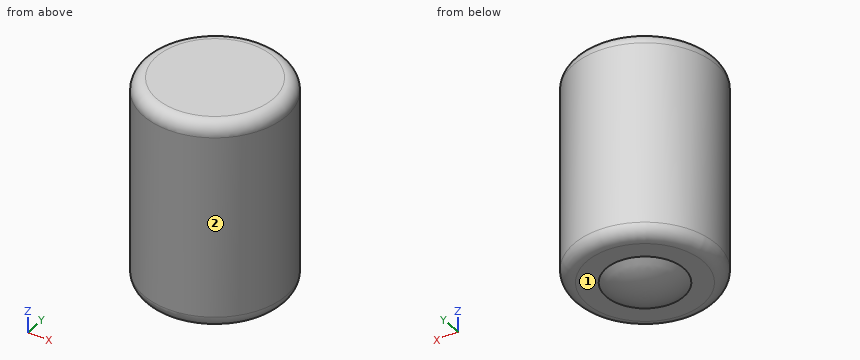
from build123d import *

# Parameters (mm, degrees)
F0_R     = 5.5
F1_DEPTH = 16
F2_R     = 1
F3_T     = -1.5
F6_R     = 1


with BuildPart() as f1:
    # F0 (on Top) → F1 (new body)
    with BuildSketch(Plane.XY):
        Circle(F0_R)
    extrude(amount=-F1_DEPTH)

    # F2
    f2_edges = [f1.edges().sort_by_distance(p)[0] for p in [
        (-5.5, 0, -16),
    ]]
    fillet(f2_edges, radius=F2_R)

    # F3 (hollow: no face is removed)
    offset(amount=F3_T, mode=Mode.SUBTRACT)

    # F4 (on Front) → F5 (revolve)
    with BuildSketch(Plane.XZ):
        with BuildLine():
            Line((3, -16), (0, -16))
            Line((0, -16), (0, -17))
            ThreePointArc((0, -17), (1.5855322487, -16.7565967462), (3, -16))
        make_face()
    revolve(axis=Axis((0, 0, -16.5), (0, 0, -1)))

    # F6
    f6_edges = [f1.edges().sort_by_distance(p)[0] for p in [
        (-5.5, 0, 0),
    ]]
    fillet(f6_edges, radius=F6_R)


solid = f1.part
Could you check a few things on this model? Use its own coordinates, in mm. Face numbers are marked on the shaded views. A direction names the side the tool comes from. Coordinates: 2 decimals unless noted, no trailing zeros. Write each loop counter-clockwise with the first axis right and the second up, starting at its lowest first coordinate (ties: lowest second). Pieces come first, ordered by that corner, then holes. Notation, with made-up numbers: (65.25, 44.5) - (108.25, 44.5) arc R25 ccw to (108.25, 56.5) - close; hole circle Ø5 at (64.25, -36). An arc over 180 degrees is marked (long way). Put each result on its own line as item: value. Start each with the question number.
Q1. I want a section at A-A on z = -12. Write out the boundary of the cut face in (x, y).
Q2. Which directions (+Z, -Z, +X, -X, +Y, -Y) give clear straight access to the entire face, cutting with the end or side of a thin tool? Please do the marked faces 1 and 2.
Q3. Please list where these lines run through material, in increasing order: L1, parallel to Y at x = 0, z = -5; L2, parallel to Z at x = -3, y = 2; L3, parallel to X at y = -1.75, z = -2.5.
Q4. I'm going to push flat-ended pins straight in: P1, Ø4.5, axis at x = 2, y = -2, coming from the -Z side; P2, Ø3, axis at x = -2.5, z = -13, coming from the +Y side; P3, Ø6.5, axis at x = 0, y = 0, coming from the +Z side; P4, Ø2, axis at x = -2, y = -0.5, coming from the -Z side. Where does each tip first touch, or does it pass through?
Checks:
1. outline: circle Ø11 at (0, 0); hole circle Ø8 at (0, 0)
2. face 1: -Z
2. face 2: +Z, -Z
3. L1: -5.5 to -4, 4 to 5.5
3. L2: -16 to -14.5, -1.5 to 0
3. L3: -5.21 to -3.6, 3.6 to 5.21
4. P1: z = -16.97
4. P2: y = 5.41
4. P3: z = 0
4. P4: z = -16.9
